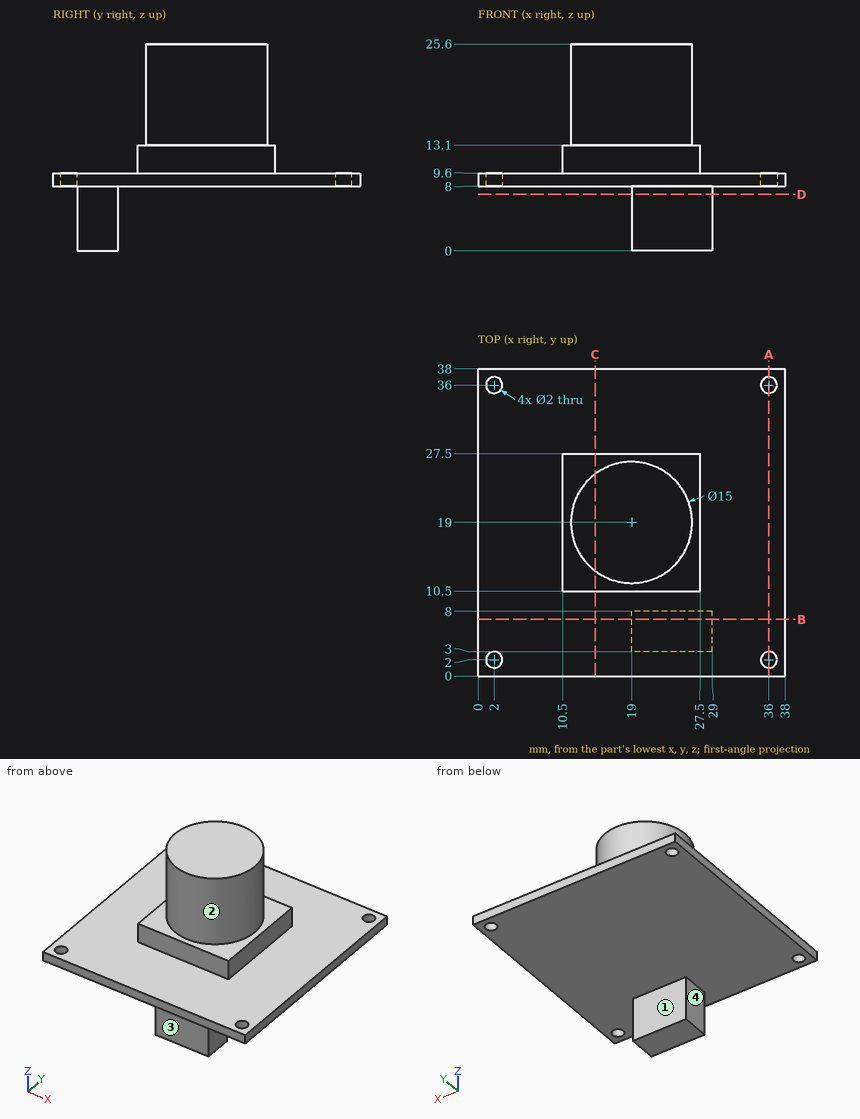
Answer from the drawing. Dimensions are ordinates in mm from the lowest x, y and z of the part. A direction names the side the tool comes from. Coordinates: 2 decimals unless noted, no trailing zeros. Loops run counter-clockwise (first coordinate to the right, second up) from the corner with the lowest first, then second, coordinate; pieces in that order, holes last. Notation, with made-up numbers: (-38.5, 41) - (2.5, 41) arc R14 ccw to (2.5, 49) - close; hole circle Ø7 at (86, 31). An arc over 180 degrees is marked (long way). Answer in a Markdown table with one row per item.
1. Find section D-D, the plane z = 7. Write down the section's boundary in (x, y), then the cut area to 3 significant figures.
Conclusion:
| item | result |
|---|---|
| outline | (19, 3) - (29, 3) - (29, 8) - (19, 8) - close |
| area | 50.0 mm² |
2. Given pin 1 (10 mm diameter, centred on x = 7.5, y = 27, fed in from -Z); pin 2 (1 mm diameter, centred on x = 19, z = 11, fed in from +Y); pin 3 (12 mm diameter, centred on y = 7.5, z = 22.5, fed in from +X); pin 4 (1.6 mm diameter, centred on x = 2, y = 2, fed in from -Z), each flat-ended and moving along its own axis, determine where each tip first touches the part or whether it passes through.
Conclusion:
| item | result |
|---|---|
| pin 1 | stops at z = 8 |
| pin 2 | stops at y = 27.5 |
| pin 3 | stops at x = 24.1 |
| pin 4 | passes through |
3. Straight lines are drawn through the part: line 1 (Y direction, x = 36, z = 8.6); line 2 (Z direction, x = 18.5, y = 8.5). For each, find the intervals that lie inside material, in ascending order.
Conclusion:
| item | result |
|---|---|
| line 1 | y = 0 to 1, 3 to 35, 37 to 38 |
| line 2 | z = 8 to 9.6 |
4. Find section A-A, the plane x = 36. Write down the section's boundary in (y, z).
Conclusion:
| item | result |
|---|---|
| outline | (0, 8) - (1, 8) - (1, 9.6) - (0, 9.6) - close; (3, 8) - (35, 8) - (35, 9.6) - (3, 9.6) - close; (37, 8) - (38, 8) - (38, 9.6) - (37, 9.6) - close |
5. Find section C-C, the plane x = 14.5. Write down the section's boundary in (y, z), then the cut area to 3 significant figures.
Conclusion:
| item | result |
|---|---|
| outline | (0, 8) - (38, 8) - (38, 9.6) - (27.5, 9.6) - (27.5, 13.1) - (25, 13.1) - (25, 25.6) - (13, 25.6) - (13, 13.1) - (10.5, 13.1) - (10.5, 9.6) - (0, 9.6) - close |
| area | 270 mm² |
6. Find section B-B, the plane y = 7. Write down the section's boundary in (x, z), then the cut area to 3 significant figures.
Conclusion:
| item | result |
|---|---|
| outline | (0, 8) - (19, 8) - (19, 0) - (29, 0) - (29, 8) - (38, 8) - (38, 9.6) - (0, 9.6) - close |
| area | 141 mm² |
7. Which of the six approach directions +Z, -Z, +X, -X, +Y, -Y give full straight-line access (tool end or side, diameter ignored) to the marked faces 1, 2, 3 and 4?
Conclusion:
| item | result |
|---|---|
| face 1 | -Z, +X, -X, +Y |
| face 2 | +Z |
| face 3 | -Z, +X, -X, -Y |
| face 4 | -Z, -X, +Y, -Y |
